Here's the drawing with two shaded views (mm, measured from the low corner). I have some questions. Round coordinates to 2 decimals unless told otherwise and drop trailing zeros. Loops run counter-clockwise (first coordinate to the right, second up) from the corner with the lowest first, then second, coordinate; pieces in that order, holes last. Notation, with made-up numbers: (10.25, -25) -> (49.25, -25) arc R21 ccw to (49.25, -12) -> close; hole circle Ø5 at (26, 68). An arc over 180 degrees is marked (long way). Write each question's results on one line, items separated by ' | '.
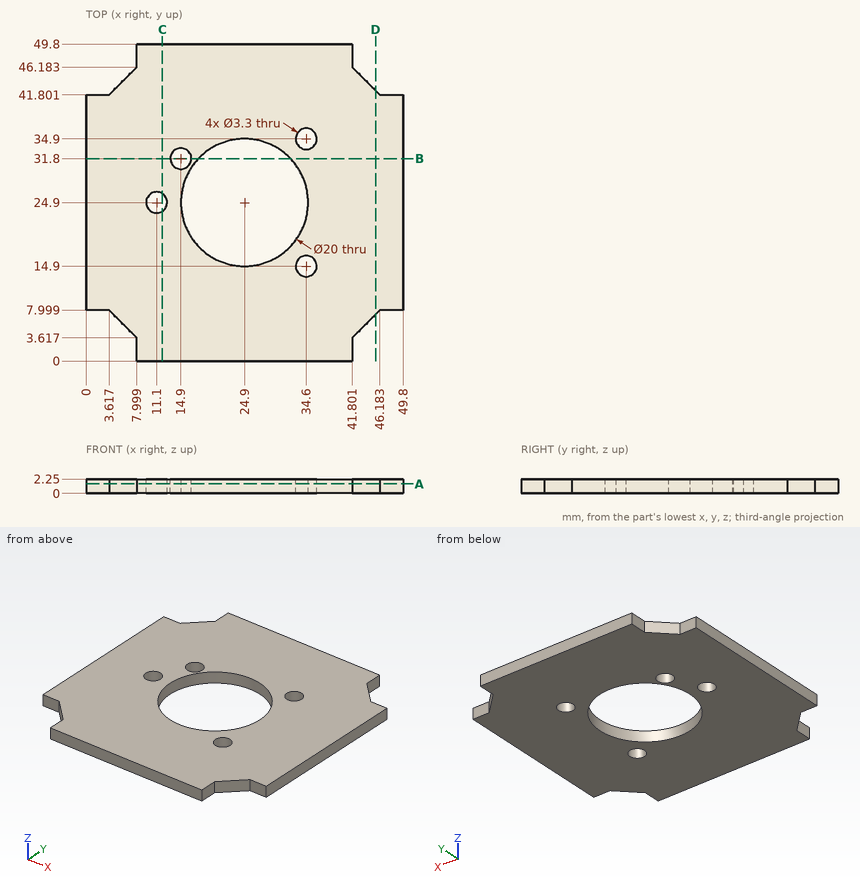
1. If we section it at B-B (y = 31.8): List the corners of the cut face in (x, z) for me.
Final values:
outline: (0, 0) -> (13.25, 0) -> (13.25, 2.25) -> (0, 2.25) -> close; (16.55, 0) -> (17.66, 0) -> (17.66, 2.25) -> (16.55, 2.25) -> close; (32.14, 0) -> (49.8, 0) -> (49.8, 2.25) -> (32.14, 2.25) -> close
2. Please list where these lines run through material, in increasing order: line 1 (X direction, y = 31.8, z = 1.05); line 2 (Y direction, x = 11.1, z = 1.65); line 3 (Y direction, x = 47.5, z = 1.05). Write a range as from..to.
Final values:
line 1: 0..13.25, 16.55..17.66, 32.14..49.8 | line 2: 0..23.25, 26.55..49.8 | line 3: 8..41.8
3. If we section it at D-D (x = 45.5): List the corners of the cut face in (y, z) for me.
Final values:
outline: (7.32, 0) -> (42.48, 0) -> (42.48, 2.25) -> (7.32, 2.25) -> close
4. Will these pins go through, and if not, where does the flat tip stop? pin 1 (0.7 mm diameter, centred on y = 48, z = 1.5, fed in from -X); pin 2 (1.1 mm diameter, centred on y = 48, z = 1, fed in from +X); pin 3 (0.7 mm diameter, centred on x = 1.5, z = 1, fed in from +Y).
Final values:
pin 1: x = 8 | pin 2: x = 41.8 | pin 3: y = 41.8
5. If we section it at C-C (x = 12): List the corners of the cut face in (y, z) for me, then the cut area to 3 significant figures.
Final values:
outline: (0, 0) -> (23.52, 0) -> (23.52, 2.25) -> (0, 2.25) -> close; (26.28, 0) -> (49.8, 0) -> (49.8, 2.25) -> (26.28, 2.25) -> close | area: 106 mm2
6. If we section it at A-A (z = 1.5): List the corners of the cut face in (x, y) for me, then the cut area to 3 significant figures.
Final values:
outline: (0, 8) -> (3.62, 8) -> (8, 3.62) -> (8, 0) -> (41.8, 0) -> (41.8, 3.62) -> (46.18, 8) -> (49.8, 8) -> (49.8, 41.8) -> (46.18, 41.8) -> (41.8, 46.18) -> (41.8, 49.8) -> (8, 49.8) -> (8, 46.18) -> (3.62, 41.8) -> (0, 41.8) -> close; hole circle Ø3.3 at (11.1, 24.9); hole circle Ø3.3 at (14.9, 31.8); hole circle Ø20 at (24.9, 24.9); hole circle Ø3.3 at (34.6, 14.9); hole circle Ø3.3 at (34.6, 34.9) | area: 1,910 mm2
